Autodesk Inventor part; units mm, degrees
ref_plane "YZ Plane" through (0, 0, 0) normal (1, 0, 0) x (0, 1, 0)
ref_plane "XZ Plane" through (0, 0, 0) normal (0, 1, 0) x (-1, 0, 0)
ref_plane "XY Plane" through (0, 0, 0) normal (0, 0, 1) x (1, 0, 0)
sketch "Sketch1" plane through (0, 0, 0) normal (0, 0, 1) x (1, 0, 0)
  line L0 (-13.5, -8.75) -> (13.5, -8.75)
  line L1 (13.5, -8.75) -> (13.5, 8.75)
  line L2 (13.5, 8.75) -> (-13.5, 8.75)
  line L3 (-13.5, 8.75) -> (-13.5, -8.75)
  line L4 (0, 0) -> (0, 8.75) construction
  line L5 (0, 0) -> (13.5, 0) construction
  circle A0 centre (0, 0) radius 4
  dimension "d0" = 27
  dimension "d2" = 8
  dimension "d3" = 17.5
extrude "Extrusion1" add sketch "Sketch1" along normal mid plane 2
properties part number "20-028Z1" material "Steel, High Strength Low Alloy"
The model under review builds one solid part; all positions refer to its coordinate system, in mm. Give positions to 0.01 mm unless a question says otherwise; leave off trailing zeros. Write each loop counter-clockwise with the first axis right and the second up, starting at its lowest first coordinate (ties: lowest second). Pieces come first, ordered by that corner, then holes. Notation, with made-up numbers: M 4.5,-11.5 L 11.5,-11.5 A8 ccw 11.5,-4.5 Z; hole C 15.25,-33.75 d9. An arc over 180 degrees is marked long. Write item = value, one per line. Start each with the question number.
Q1. For line 1 (Y direction, x = 0, z = -0.5); line 2 (X direction, y = -2.5, z = -0.35); line 3 (X direction, y = -0.25, z = 0.5), list the stretches that pass through material, from the lowest coordinate up.
Q2. Clearance check with a flat-ended pin moving along its axis: pin 1 (6.5 mm diameter, centred on x = 0, y = 0, fed in from -Z). State where the tip first meets the part, or that it passes through.
Q3. We need section C-C (z = 0.4). State the section outline as (x, y) points, plus the area to 3 significant figures.
Q4. We need section A-A (y = 0). State the section outline as (x, z) points, plus the area to 3 significant figures.
Q5. Mouldability with a two-part tool opening along Y and no side actions: class faces 1 (the face through (0, 8.75, 0)), 2 (the face through (3, 4, 1)), 3 (the face through (-0.867, 3.905, -0.014)) as released by +Y, released by -Y, zero draft, split by the parting line, or undercut.
Q6. We need section B-B (x = 0). State the section outline as (y, z) points.
Result set:
q1.line_1 = -8.75 to -4, 4 to 8.75
q1.line_2 = -13.5 to -3.12, 3.12 to 13.5
q1.line_3 = -13.5 to -3.99, 3.99 to 13.5
q2.pin_1 = through
q3.outline = M -13.5,-8.75 L 13.5,-8.75 L 13.5,8.75 L -13.5,8.75 Z; hole C 0,0 d8
q3.area = 422 mm2
q4.outline = M -13.5,-1 L -4,-1 L -4,1 L -13.5,1 Z; M 4,-1 L 13.5,-1 L 13.5,1 L 4,1 Z
q4.area = 38.0 mm2
q5.face_1 = released by +Y
q5.face_2 = zero draft
q5.face_3 = undercut
q6.outline = M -8.75,-1 L -4,-1 L -4,1 L -8.75,1 Z; M 4,-1 L 8.75,-1 L 8.75,1 L 4,1 Z
